Read the model definition and answer for the solid it produces. Units are mm, in the model's axes. Round coordinates to 2 decimals unless told otherwise and drop trailing zeros. Write each loop counter-clockwise with the first axis right and the second up, starting at its lowest first coordinate (ties: lowest second). Pieces come first, ordered by that corner, then holes. Notation, with made-up numbers: (36, -17.75) -> (60, -17.75) arc R24 cw to (60, 21.25) -> close; hole circle Ø4 at (-20.5, 38.5). An arc over 180 degrees is marked (long way). Return JSON: item names as keys, results as strings.
from build123d import *

# Parameters (mm, degrees)
SKETCH1_W           = 1219.2
SKETCH1_H           = 914.4
BOSS_EXTRUDE1_DEPTH = 18.25625
SKETCH2_W           = 203.2
SKETCH2_H           = 101.6
CUT_EXTRUDE1_DEPTH  = 933.742714077
FILLET1_R           = 12.7


with BuildPart() as part:
    # Sketch1 → Boss-Extrude1 (new body)
    with BuildSketch(Plane.XY):
        with Locations((203.2, 0)):
            Rectangle(SKETCH1_W, SKETCH1_H)
    extrude(amount=BOSS_EXTRUDE1_DEPTH)

    # Sketch2 → Cut-Extrude1 (cut, through all)
    with BuildSketch(Plane.XY.offset(18.25625)):
        with Locations((203.2, -382.699600817)):
            Rectangle(SKETCH2_W, SKETCH2_H)
    extrude(amount=-CUT_EXTRUDE1_DEPTH, mode=Mode.SUBTRACT)

    # Fillet1
    fillet1_edges = [part.edges().sort_by_distance(p)[0] for p in [
        (101.6, -433.499600817, 9.128125),
        (101.6, -331.899600817, 9.128125),
        (304.8, -331.899600817, 9.128125),
        (304.8, -433.499600817, 9.128125),
    ]]
    fillet(fillet1_edges, radius=FILLET1_R)


solid = part.part
Item 1: Section A-A (x = 225) is taken. Give the vertices of the cut face in (y, z), then the cut area to 3 significant figures.
Worked answers:
{"outline": "(-457.2, 0) -> (-433.5, 0) -> (-433.5, 18.26) -> (-457.2, 18.26) -> close; (-331.9, 0) -> (457.2, 0) -> (457.2, 18.26) -> (-331.9, 18.26) -> close", "area": "14,800 mm2"}
Item 2: Section B-B (z = 6) is taken. Give the vertices of the cut face in (x, y), then the cut area to 3 significant figures.
Worked answers:
{"outline": "(-406.4, -457.2) -> (812.8, -457.2) -> (812.8, 457.2) -> (-406.4, 457.2) -> close; hole (101.6, -420.8) arc R12.7 ccw to (114.3, -433.5) -> (292.1, -433.5) arc R12.7 ccw to (304.8, -420.8) -> (304.8, -344.6) arc R12.7 ccw to (292.1, -331.9) -> (114.3, -331.9) arc R12.7 ccw to (101.6, -344.6) -> close", "area": "1,090,000 mm2"}
Item 3: Straight lines are drawn through the part: L1, parallel to Y at x = 157.5, z = 11.25; L2, parallel to Y at x = 112, z = 2.75; L3, parallel to X at y = -348.5, z = 16. For each, find the intervals that lie inside material, in ascending order. Write a range as [from, to].
Worked answers:
{"L1": "y = [-457.2, -433.5], [-331.9, 457.2]", "L2": "y = [-457.2, -433.29], [-332.11, 457.2]", "L3": "x = [-406.4, 101.6], [304.8, 812.8]"}
